from build123d import *

# Parameters (mm, degrees)
F1_DEPTH = 25.4
F2_DEPTH = 76.2
F3_R     = 12.7
F4_DEPTH = 76.201
F6_DEPTH = 25.401


with BuildPart() as f1:
    # F0 (on Top) → F1 (new body)
    with BuildSketch(Plane.XY):
        with BuildLine():
            Line((54.951176, 25.445276), (-49.537972, 25.445276))
            ThreePointArc((-49.537972, 25.445276), (-26.458922, 0.186695), (-49.224562, -25.354724))
            Line((-49.224562, -25.354724), (54.951176, -25.354724))
            ThreePointArc((54.951176, -25.354724), (76.688998, 0.045276), (54.951176, 25.445276))
        make_face()
    extrude(amount=F1_DEPTH)

    # F0 (on Top) → F2 (join)
    with BuildSketch(Plane.XY):
        with BuildLine():
            Line((-49.537972, 25.445276), (-54.447679, 25.445276))
            ThreePointArc((-54.447679, 25.445276), (-73.704644, 0.163115), (-54.761089, -25.354724))
            Line((-54.761089, -25.354724), (-49.224562, -25.354724))
            ThreePointArc((-49.224562, -25.354724), (-26.458922, 0.186695), (-49.537972, 25.445276))
        make_face()
    extrude(amount=F2_DEPTH)

    # F3 (on face) → F4 (cut, through all)
    with BuildSketch(Plane.XY.offset(76.2)):
        with Locations((-51.992825, 0.029164)):
            Circle(F3_R)
    extrude(amount=-F4_DEPTH, mode=Mode.SUBTRACT)

    # F5 (on face) → F6 (cut, through all)
    with BuildSketch(Plane.XY.offset(25.4)):
        with BuildLine():
            Line((49.735157, 11.921302), (-1.064843, 11.921302))
            ThreePointArc((-1.064843, 11.921302), (-13.764843, -0.778698), (-1.064843, -13.478698))
            Line((-1.064843, -13.478698), (49.735157, -13.478698))
            ThreePointArc((49.735157, -13.478698), (62.435157, -0.778698), (49.735157, 11.921302))
        make_face()
    extrude(amount=-F6_DEPTH, mode=Mode.SUBTRACT)


solid = f1.part
The listing builds one solid part. Answer for the finished solid, in the listing's coordinates (mm). A direction names the side the tool comes from. Round coordinates to 2 decimals unless told otherwise and drop trailing zeros. Order: outer loops, then holes, each group sorted by start corner. A loop starts at its lowest first (then second) coordinate and runs counter-clockwise, first axis right, second up. Notation, with made-up numbers: (37.25, 25.25) -> (79.25, 25.25) arc R18 ccw to (79.25, 46.25) -> close; hole circle Ø9 at (39.5, -25.5). An arc over 180 degrees is marked (long way). Write each question's results on one line, items separated by ' | '. Start each with the question number.
Q1. Each of these flat-tipped pins is pushed along its axis until it touches: pin 1 (8 mm diameter, centred on y = -12.5, z = 48.5, fed in from +X); pin 2 (10 mm diameter, centred on y = 17, z = 37.5, fed in from -X); pin 3 (5 mm diameter, centred on y = 4, z = 23, fed in from -X). Where does it stop, or does it pass through?
Q2. Find section D-D (x = -44.5). Determine the outline of the cut face in (y, z), then the cut area to 3 significant figures.
Q3. Which of the six approach directions +Z, -Z, +X, -X, +Y, -Y give full straight-line access (tool end or side, diameter ignored) to faces 1 (the flat face through (-40, -5, 76.2)), 2 (the cylindrical face through (-26.46, -0.34, 50.44)), 3 (the cylindrical face through (-13.76, -0.5, 12.88))?
Q4. The mould has two halves that part along Y. Classify faces 4 (the cylindrical face through (-73.7, 0.6, 37.6)), 5 (the flat face through (27, 17, 25.4)), 6 (the cylindrical face through (-62.07, -7.7, 38.63)): pulls with the +Y half, pulls with the -Y half, needs draft (parallel to the pull), parting line crosses it, or undercut.
Q5. Find section B-B (y = 2). Determine the outline of the cut face in (x, z).
Q6. Find section C-C (z = 20). Determine the outline of the cut face in (x, y), then the cut area to 3 significant figures.
Q7. Find section A-A (x = 15). Determine the outline of the cut face in (y, z).
Q8. Straight lines are drawn through the part: probe 1 along Y at (x, z) = (-52.5, 37); probe 2 along Y at (x, z) = (37, 24); probe 3 along X at (y, z) = (4.5, 3). For each, find the intervals that lie inside material, in ascending order. Write a range as from..to.
Worked answers:
1) pin 1: stops at x = -27.93 | pin 2: stops at x = -70.83 | pin 3: stops at x = -73.66
2) outline: (-25.35, 0) -> (-10.22, 0) -> (-10.22, 76.2) -> (-24.38, 76.2) -> (-24.38, 25.4) -> (-25.35, 25.4) -> close; (10.28, 0) -> (25.45, 0) -> (25.45, 25.4) -> (24.44, 25.4) -> (24.44, 76.2) -> (10.28, 76.2) -> close | area: 2,210 mm2
3) face 1: +Z, +X, -X, +Y, -Y | face 2: +Z, +X | face 3: +Z, -Z
4) face 4: parting line crosses it | face 5: needs draft | face 6: undercut
5) outline: (-73.63, 0) -> (-64.54, 0) -> (-64.54, 76.2) -> (-73.63, 76.2) -> close; (-39.45, 0) -> (-13.46, 0) -> (-13.46, 25.4) -> (-26.53, 25.4) -> (-26.53, 76.2) -> (-39.45, 76.2) -> close; (62.13, 0) -> (76.61, 0) -> (76.61, 25.4) -> (62.13, 25.4) -> close
6) outline: (-54.76, -25.35) -> (54.95, -25.35) arc R25.71 ccw to (54.95, 25.45) -> (-54.45, 25.45) arc R26.44 ccw to start; hole circle Ø25.4 at (-51.99, 0.03); hole (-1.06, -13.48) -> (49.74, -13.48) arc R12.7 ccw to (49.74, 11.92) -> (-1.06, 11.92) arc R12.7 ccw to start | area: 4,810 mm2
7) outline: (-25.35, 0) -> (-13.48, 0) -> (-13.48, 25.4) -> (-25.35, 25.4) -> close; (11.92, 0) -> (25.45, 0) -> (25.45, 25.4) -> (11.92, 25.4) -> close
8) probe 1: y = -25.35..-12.66, 12.72..25.45 | probe 2: y = -25.35..-13.48, 11.92..25.45 | probe 3: x = -73.32..-63.88, -40.11..-12.62, 61.29..76.3
